```python
from build123d import *

# Parameters (mm, degrees)
SKETCH_1_R          = 1.75
SKETCH_1_R_2        = 3
EXTRUDE_1_DEPTH     = 3
CUT_EXTRUDE_2_DEPTH = 10
SKETCH_5_R          = 1.55
CUT_EXTRUDE_3_DEPTH = 10


with BuildPart() as part:
    # 草图1 → 凸台-拉伸1 (new body)
    with BuildSketch(Plane.XY):
        Polygon((65, -25), (65, 75.163369284), (44.840227583, 105), (-44.840227583, 105), (-65, 75.163369284), (-65, -25), (-65, -35), (65, -35), align=None)
        with Locations((44.25, -15)):
            Circle(SKETCH_1_R, mode=Mode.SUBTRACT)
        with Locations((20.25, -15)):
            Circle(SKETCH_1_R, mode=Mode.SUBTRACT)
        with Locations((20.25, 15)):
            Circle(SKETCH_1_R, mode=Mode.SUBTRACT)
        with Locations((44.25, 15)):
            Circle(SKETCH_1_R, mode=Mode.SUBTRACT)
        with Locations(Location((-44.25, 15, 0), (0, 0, 180))):
            Circle(SKETCH_1_R, mode=Mode.SUBTRACT)
        with Locations(Location((-20.25, 15, 0), (0, 0, 180))):
            Circle(SKETCH_1_R, mode=Mode.SUBTRACT)
        with Locations(Location((-20.25, -15, 0), (0, 0, 180))):
            Circle(SKETCH_1_R, mode=Mode.SUBTRACT)
        with Locations(Location((-44.25, -15, 0), (0, 0, 180))):
            Circle(SKETCH_1_R, mode=Mode.SUBTRACT)
        with Locations((-17.5, 95)):
            Circle(SKETCH_1_R_2, mode=Mode.SUBTRACT)
        with Locations(Location((17.5, 95, 0), (0, 0, 180))):
            Circle(SKETCH_1_R_2, mode=Mode.SUBTRACT)
        with Locations((-17.5, 50)):
            Circle(SKETCH_1_R_2, mode=Mode.SUBTRACT)
        with Locations(Location((17.5, 50, 0), (0, 0, 180))):
            Circle(SKETCH_1_R_2, mode=Mode.SUBTRACT)
        with BuildLine():
            Line((-10, 40), (10, 40))
            ThreePointArc((10, 40), (11.5, 38.5), (10, 37))
            Line((10, 37), (-10, 37))
            ThreePointArc((-10, 37), (-11.5, 38.5), (-10, 40))
        make_face(mode=Mode.SUBTRACT)
        with BuildLine():
            Line((-10, -18), (10, -18))
            ThreePointArc((10, -18), (11.5, -19.5), (10, -21))
            Line((10, -21), (-10, -21))
            ThreePointArc((-10, -21), (-11.5, -19.5), (-10, -18))
        make_face(mode=Mode.SUBTRACT)
    extrude(amount=EXTRUDE_1_DEPTH)

    # 草图3 → 切除-拉伸2 (cut)
    with BuildSketch(Plane(origin=(0, 0, 0), x_dir=(-1, 0, 0), z_dir=(0, 0, -1))):
        with BuildLine():
            Line((-9.52, -27), (-9.52, -24))
            ThreePointArc((-9.52, -24), (-8, -22.48), (-6.48, -24))
            Line((-6.48, -24), (-6.48, -27))
            ThreePointArc((-6.48, -27), (-8, -28.52), (-9.52, -27))
        make_face()
        with BuildLine():
            Line((9.52, -27), (9.52, -24))
            ThreePointArc((9.52, -24), (8, -22.48), (6.48, -24))
            Line((6.48, -24), (6.48, -27))
            ThreePointArc((6.48, -27), (8, -28.52), (9.52, -27))
        make_face()
    extrude(amount=-CUT_EXTRUDE_2_DEPTH, mode=Mode.SUBTRACT)

    # 草图5 → 切除-拉伸3 (cut)
    with BuildSketch(Plane.XY.offset(3)):
        with Locations((-47.5, 70)):
            Circle(SKETCH_5_R)
        with Locations((47.5, 70)):
            Circle(SKETCH_5_R)
        with Locations((-47.5, -25)):
            Circle(SKETCH_5_R)
        with Locations((47.5, -25)):
            Circle(SKETCH_5_R)
    extrude(amount=-CUT_EXTRUDE_3_DEPTH, mode=Mode.SUBTRACT)


solid = part.part
```
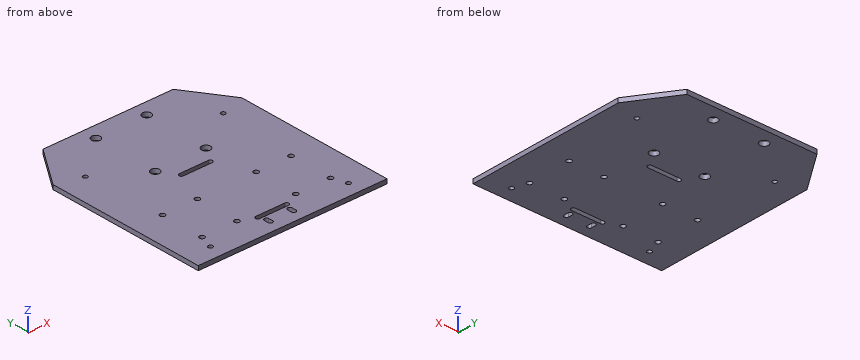
Here's how the part is built. I have some questions about the finished solid (model axes, mm). Coordinates: 2 decimals unless noted, no trailing zeros. Order: outer loops, then holes, each group sorted by start corner. A loop starts at its lowest first (then second) coordinate and runs counter-clockwise, first axis right, second up.
1) Imagine slicing it at C-C on y = 87. List the corners of the cut face in (x, z) for me, and give its area (3 significant figures).
2) Imagine slicing it at B-B on x = 54. List the corners of the cut face in (y, z) for me, and give its area (3 significant figures).
3) I need wall thicknesses on line 1 (Y direction, x = -17.5, z = 2.4); line 2 (Y direction, x = -6, z = 1); line 3 (X direction, y = 70, z = 1.3). Which ranges of each line are inside material? Lowest first, please.
4) Imagine slicing it at A-A on z = 1. State how many separate pieces and enclosed holes the cut face has, and give its area (3 significant figures).
Response values:
1. outline: (-57, 0) - (57, 0) - (57, 3) - (-57, 3) - close
1. area: 342 mm2
2. outline: (-35, 0) - (91.44, 0) - (91.44, 3) - (-35, 3) - close
2. area: 379 mm2
3. line 1: y = -35 to 47, 53 to 92, 98 to 105
3. line 2: y = -35 to -21, -18 to 37, 40 to 105
3. line 3: x = -65 to -49.05, -45.95 to 45.95, 49.05 to 65
4. separate pieces: 1
4. enclosed holes: 20
4. area: 17,200 mm2
